from build123d import *

# Parameters (mm, degrees)
SKETCH2_R           = 5
BOSS_EXTRUDE1_DEPTH = 7
BOSS_EXTRUDE2_DEPTH = 12.5


with BuildPart() as part:
    # Sketch2 → Boss-Extrude1 (new body)
    with BuildSketch(Plane(origin=(0, 0, 0), x_dir=(1, 0, 0), z_dir=(0, 1, 0))):
        with Locations(Location((0, 0, 0), (0, 0, 270))):
            Circle(SKETCH2_R)
    extrude(amount=BOSS_EXTRUDE1_DEPTH)

    # Sketch3 → Boss-Extrude2 (add)
    with BuildSketch(Plane(origin=(0, 7, 0), x_dir=(1, 0, 0), z_dir=(0, 1, 0))):
        with BuildLine():
            Line((-3.975, 2.99165506), (-3.975, -2.99165506))
            ThreePointArc((-3.975, -2.99165506), (0, -4.975), (3.975, -2.99165506))
            Line((3.975, -2.99165506), (3.975, 2.99165506))
            ThreePointArc((3.975, 2.99165506), (0, 4.975), (-3.975, 2.99165506))
        make_face()
    extrude(amount=BOSS_EXTRUDE2_DEPTH)


solid = part.part
For this review, take the finished solid that the model builds, in its own axes (mm). A direction names the side the tool comes from. Give positions to 0.01 mm unless a question says otherwise; leave off trailing zeros. Loops run counter-clockwise (first coordinate to the right, second up) from the corner with the lowest first, then second, coordinate; pieces in that order, holes last. Notation, with made-up numbers: (-22.5, 68.5) -> (-7.5, 68.5) arc R23 ccw to (-7.5, 83.5) -> close; hole circle Ø2 at (54, -39). An arc over 180 degrees is marked (long way). One line per question, with ' | ' between items.
1) For faces 1 (the cylindrical face through (0.064, 13.162, -4.975)), 2 (the cylindrical face through (-0.064, 13.162, 4.975)), 3 (the flat face through (-3.975, 13, 0)), 4 (the flat face through (3.975, 13, 0)), 5 (the flat face through (0, 19.5, 0)), list the 3-axis set-ups (+Z, -Z, +X, -X, +Y, -Y) from which the entire face can be reached by the end or side of a thin tool; tool diameter is ignored.
Resolved:
face 1: -Z, +Y | face 2: +Z, +Y | face 3: +Z, -Z, -X, +Y | face 4: +Z, -Z, +X, +Y | face 5: +Z, -Z, +X, -X, +Y
2) We need section A-A (z = 0). Write out the cut boundary in (x, y) (3 decimals), plus the area to 3 significant figures.
Resolved:
outline: (-5, 0) -> (5, 0) -> (5, 7) -> (3.975, 7) -> (3.975, 19.5) -> (-3.975, 19.5) -> (-3.975, 7) -> (-5, 7) -> close | area: 169 mm2
3) We need section C-C (y = 3.75). Write out the cut boundary in (x, z), plus the area to 3 significant figures.
Resolved:
outline: circle Ø10 at (0, 0) | area: 78.5 mm2
4) To check wall thickness, follow probe 1 along X at (y, z) = (10.5, 2.75) (3 decimals); probe 2 along X at (y, z) = (1.5, 3.75); probe 3 along Z at (x, y) = (-1.5, 15.25). State the ranges of each line that lie inside material, in increasing order.
Resolved:
probe 1: x = -3.975 to 3.975 | probe 2: x = -3.31 to 3.31 | probe 3: z = -4.74 to 4.74
5) Insertion check: pin 1 Ø1 at (y, z) = (9.5, 0.5) entering from +X (3 decimals); pin 2 Ø5 at (y, z) = (11, -1) entering from -X (3 decimals). Each pin has a flat end and moves straight along its axis. Give the tip position at first contact, or say it passes through.
Resolved:
pin 1: stops at x = 3.975 | pin 2: stops at x = -3.975
6) We need section D-D (y = 9.75). Write out the cut boundary in (x, z) (3 decimals), plus the area to 3 significant figures.
Resolved:
outline: (-3.975, -2.992) arc R4.975 ccw to (3.975, -2.992) -> (3.975, 2.992) arc R4.975 ccw to (-3.975, 2.992) -> close | area: 69.6 mm2
